Autodesk Inventor part; units mm, degrees
ref_plane "YZ Plane" through (0, 0, 0) normal (1, 0, 0) x (0, 1, 0)
ref_plane "XZ Plane" through (0, 0, 0) normal (0, 1, 0) x (-1, 0, 0)
ref_plane "XY Plane" through (0, 0, 0) normal (0, 0, 1) x (1, 0, 0)
sketch "Sketch1" plane through (0, 0, 0) normal (0, 0, 1) x (1, 0, 0)
  line L0 (0, 0) -> (25, 0)
  line L1 (25, 0) -> (25, 40)
  line L2 (25, 40) -> (0, 40)
  line L3 (0, 40) -> (0, 0)
  dimension "d1" = 25
  dimension "d2" = 40
  dimension "d3" = 25
extrude "Extrusion1" add sketch "Sketch1" against normal blind 30
sketch "Sketch2" plane through (25, 0, 0) normal (1, 0, 0) x (0, 0, -1)
  line L0 (0, 0) -> (30, 0)
  circle A0 centre (15, 6.56) radius 2.46
extrude "Extrusion2" cut sketch "Sketch2" against normal blind 30
sketch "Sketch3" plane through (0, 0, 0) normal (-1, 0, 0) x (0, 0, 1)
  line L0 (0, 0) -> (-30, 0)
  line L1 (-25.05, 0) -> (-4.95, 0)
  line L2 (-4.95, 0) -> (-4.95, 33.12)
  line L3 (-4.95, 33.12) -> (-25.05, 33.12)
  line L4 (-25.05, 33.12) -> (-25.05, 0)
  dimension "d11" = 20.1
extrude "Extrusion3" cut sketch "Sketch3" against normal blind 20
sketch "Sketch4" plane through (0, 0, 0) normal (0, -1, 0) x (1, 0, 0)
  line L0 (20, -4.95) -> (20, -25.05)
  line L1 (20, -15) -> (25, -15)
  line L2 (25, 0) -> (25, -30)
  line L3 (20, -8.025) -> (25, -8.025)
  line L4 (25, -8.025) -> (25, -21.975)
  line L5 (25, -21.975) -> (20, -21.975)
  line L6 (20, -21.975) -> (20, -8.025)
  line L7 (20, -8.025) -> (25, -21.975) construction
  line L8 (25, -8.025) -> (20, -21.975) construction
  line L9 (25, -12.54) -> (25, -17.46)
  point P0 (0, 0)
  point P1 (22.5, -15)
  dimension "d14" = 13.95
extrude "Extrusion4" add sketch "Sketch4" along normal blind 15
sketch "Sketch5" plane through (20, 0, 0) normal (-1, 0, 0) x (0, 0, 1)
  circle A0 centre (-15, 6.56) radius 2.46
  circle A1 centre (-15, 6.56) radius 4.7025
  circle A2 centre (-15, 6.56) radius 2.46
  circle A3 centre (-15, 6.56) radius 2.46
  point P0 (0, 0)
  dimension "d17" = 9.405
extrude "Extrusion5" cut sketch "Sketch5" against normal blind 2.1
sketch "Sketch6" plane through (25, 0, 0) normal (1, 0, 0) x (0, 0, -1)
  circle A0 centre (15, 6.56) radius 4.7025
  line L0 (15, 6.56) -> (15, 23.56)
  circle A1 centre (15, 23.56) radius 2.46
  point P0 (0, 0)
  dimension "d20" = 17
  dimension "d21" = 4.92
extrude "Extrusion6" cut sketch "Sketch6" against normal blind 10 contours A1
sketch "Sketch7" plane through (20, 0, 0) normal (-1, 0, 0) x (0, 0, 1)
  circle A0 centre (-15, 23.56) radius 2.46
  circle A1 centre (-15, 23.56) radius 4.7025
  point P0 (0, 0)
  dimension "d24" = 9.405
extrude "Extrusion7" cut sketch "Sketch7" against normal blind 2.1
sketch "Sketch9" plane through (25, 0, 0) normal (1, 0, 0) x (0, 0, -1)
  circle A0 centre (15, 6.56) radius 2.46
  circle A1 centre (15, 6.56) radius 2.46
  circle A2 centre (15, 23.56) radius 2.46
  circle A3 centre (15, 23.56) radius 2.46
  line L0 (30, 40) -> (30, 0)
  line L1 (30, 0) -> (30, 40)
  line L2 (30, 40) -> (0, 40)
  line L3 (0, 40) -> (0, 0)
  line L4 (0, 0) -> (8.025, 0)
  line L5 (21.975, 0) -> (21.975, -15)
  line L6 (21.975, -15) -> (8.025, -15)
  line L7 (8.025, -15) -> (8.025, 0)
  line L8 (0, 0) -> (8.025, 0)
  line L9 (21.975, 0) -> (30, 0)
extrude "Extrusion8" add sketch "Sketch9" along normal blind 5
sketch "Sketch10" plane through (0, 40, 0) normal (0, 1, 0) x (1, 0, 0)
  line L0 (0, 30) -> (30, 30)
  line L1 (30, 0) -> (0, 0)
  line L2 (0, 30) -> (30, 30)
  line L3 (30, 30) -> (30, 0)
  line L4 (30, 0) -> (0, 0)
  line L5 (0, 0) -> (0, 30)
extrude "Extrusion9" add sketch "Sketch10" along normal blind 30
sketch "Sketch12" plane through (30, 0, 0) normal (1, 0, 0) x (0, 0, -1)
  circle A0 centre (15, 6.56) radius 2.46
  line L0 (15, 6.56) -> (15, 15.06)
  circle A1 centre (15, 15.06) radius 2.525
  point P0 (0, 0)
  dimension "d31" = 8.5
  dimension "d33" = 5.05
extrude "Extrusion10" cut sketch "Sketch12" against normal blind 30 contours A1
sketch "Sketch14" plane through (0, 0, 0) normal (0, 0, 1) x (1, 0, 0)
  line L0 (30, 70) -> (0, 70)
  line L1 (0, 70) -> (0, 85)
  line L2 (-15, 100) -> (-23, 100)
  line L3 (30, 0) -> (30, 70)
  line L4 (30, 113) -> (30, 70)
  arc A0 (0, 85) -> (-15, 100) centre (-15, 85) ccw
  line L5 (30, 105) -> (30, 100)
  line L6 (-23, 128) -> (15, 128)
  line L7 (30, 113) -> (15, 128)
  line L8 (-23, 128) -> (-23, 100)
  point P0 (0, 0)
  point P1 (0, 100)
  dimension "d47" = 30
  dimension "d54" = 15
  dimension "d69" = 28
extrude "Extrusion12" add sketch "Sketch14" against normal blind 30
sketch "Sketch15" plane through (0, 0, -25.05) normal (-1, 0, 0) x (0, 0, 1)
  line L0 (0, 33.12) -> (20.1, 33.12)
  line L1 (20.1, 33.12) -> (20.1, 0)
  line L2 (0, 33.12) -> (20.1, 33.12)
  line L3 (20.1, 33.12) -> (20.1, 31.1)
  line L4 (20.1, 31.1) -> (0, 31.1)
  line L5 (0, 31.1) -> (0, 33.12)
  point P0 (25.05, 0)
  dimension "d57" = 2.02
extrude "Extrusion13" add sketch "Sketch15" against normal blind 20
sketch "Sketch21" plane through (-23, 128, 0) normal (0, 1, 0) x (1, 0, 0)
  line L0 (0, 0) -> (0, 30)
  line L1 (0, 15) -> (0, 5)
  line L2 (0, 25) -> (0, 15)
  line L3 (0, 25) -> (5, 15)
  line L4 (5, 15) -> (0, 5)
  point P0 (23, 0)
  dimension "d82" = 10
extrude "Extrusion15" cut sketch "Sketch21" against normal through all
properties part number "orien_b_15mm"
Can you work these out from the model? Positions are in its coordinate system, mm. A direction names the side the tool comes from. Coordinates: 2 decimals unless noted, no trailing zeros. Order: outer loops, then holes, each group sorted by start corner. A loop starts at its lowest first (then second) coordinate and runs counter-clockwise, first axis right, second up.
1. I need wall thicknesses on line 1 (Y direction, x = 27.5, z = -15) (3 decimals); line 2 (Z direction, x = 25.5, y = 6.56); line 3 (Y direction, x = 28.5, z = -15) (3 decimals). Which ranges of each line are inside material? Lowest first, please.
2. If we section it at C-C (x = 11.5): Please give me the cut outline in (y, z), then the cut area to 3 significant figures.
3. For faces 1 (the face through (10, 16, -25.05)), 2 (the face through (-20.535, 114.196, -20.07)), 3 (the face through (-17, 100, -15)), 4 (the face through (18, 0, -27)), which set-ups out of +Z, -Z, +X, -X, +Y, -Y let a thin tool reach every point of the face, with its end or its side?
4. If we section it at B-B (x = 26.5): Please give me the cut outline in (y, z) (3 decimals), then the cut area to 3 significant figures.
5. If we section it at D-D (y = 40): Please give me the cut outline in (x, z).
6. I'm going to push flat-ended pins straight in: pin 1 (3 mm diameter, centred on y = 23.56, z = -15, fed in from -X); pin 2 (5 mm diameter, centred on y = 86.5, z = -23.5, fed in from -X); pin 3 (4 mm diameter, centred on x = 7.5, z = -22, fed in from -Y); pin 4 (16 mm diameter, centred on x = 10, z = -11, fed in from -Y). Where does each tip first touch, or does it pass through?
7. Thinking about a two-plate mould opening in Y: for faces 5 (the face through (25.995, 7.502, -17.272)), 6 (the face through (-4, 128, -15)), 7 (the face through (9, 65, 0)), which applies, +Y half, -Y half, draft (parallel to the pull), parting line (faces both ways), or undercut?
8. If we section it at A-A (y = 15.06): Please give me the cut outline in (x, z) (3 decimals).
Entries:
1. line 1: y = -15 to 4.1, 9.02 to 12.535, 17.585 to 21.1, 26.02 to 115.5
1. line 2: z = -30 to -17.46, -12.54 to 0
1. line 3: y = -15 to 4.1, 9.02 to 12.535, 17.585 to 21.1, 26.02 to 114.5
2. outline: (0, -30) - (128, -30) - (128, 0) - (0, 0) - (0, -4.95) - (31.1, -4.95) - (31.1, -25.05) - (0, -25.05) - close
2. area: 3,210 mm2
3. face 1: -X, -Y
3. face 2: -X, +Y, -Y
3. face 3: +Z, -Z, -X, -Y
3. face 4: -Z, +X, -X, -Y
4. outline: (-15, -21.975) - (0, -21.975) - (0, -30) - (116.5, -30) - (116.5, 0) - (0, 0) - (0, -8.025) - (-15, -8.025) - close; hole circle Ø4.92 at (6.56, -15); hole circle Ø5.05 at (15.06, -15); hole circle Ø4.92 at (23.56, -15)
4. area: 3,650 mm2
5. outline: (0, -30) - (30, -30) - (30, 0) - (0, 0) - close
6. pin 1: passes through
6. pin 2: stops at x = -0.54
6. pin 3: stops at y = 31.1
6. pin 4: stops at y = 0
7. face 5: undercut
7. face 6: +Y half
7. face 7: draft
8. outline: (0, -30) - (30, -30) - (30, -17.525) - (20, -17.525) - (20, -25.05) - (0, -25.05) - close; (0, -4.95) - (20, -4.95) - (20, -12.475) - (30, -12.475) - (30, 0) - (0, 0) - close
